```python
from build123d import *

# Parameters (mm, degrees)
SKETCH_1_R               = 3
PLUNGER_1_DEPTH          = 7.4
SKETCH_2_R               = 4.5
RETENTION_FLANGE_2_DEPTH = 1.2


with BuildPart() as part:
    # Эскиз1 → Plunger_1 (new body)
    with BuildSketch(Plane(origin=(0, -68, 0), x_dir=(1, 0, 0), z_dir=(0, 1, 0))):
        with Locations(Location((38, -77, 0), (0, 0, 270))):
            Circle(SKETCH_1_R)
    extrude(amount=PLUNGER_1_DEPTH)

    # Эскиз2 → Retention_flange_2 (add)
    with BuildSketch(Plane(origin=(0, -63.8, 0), x_dir=(1, 0, 0), z_dir=(0, 1, 0))):
        with Locations(Location((38, -77, 0), (0, 0, 270))):
            Circle(SKETCH_2_R)
    extrude(amount=RETENTION_FLANGE_2_DEPTH)


solid = part.part
```
Geometry check sheet. Reference: the model listing, model coordinates, mm. A direction names the side the tool comes from. Give positions to 0.01 mm unless a question says otherwise; leave off trailing zeros. Write each loop counter-clockwise with the first axis right and the second up, starting at its lowest first coordinate (ties: lowest second). Pieces come first, ordered by that corner, then holes. Notation, with made-up numbers: (29, 13) -> (37, 13) arc R21 ccw to (37, 40) -> close; hole circle Ø3 at (30, 28.25). An arc over 180 degrees is marked (long way). Use one line per item in the form item = value.
Item 1: Sectioned sample at C-C on y = -67. Enter the section's corners in (x, z), plus the area to 3 significant figures.
Results list:
outline = circle Ø6 at (38, 77)
area = 28.3 mm2
Item 2: Scan lines: line 1 (Y direction, x = 39, z = 80.75); line 2 (Z direction, x = 38, y = -62.25); line 3 (X direction, y = -61.25, z = 78.75). Record each from-to range of solid material in increasing order.
Results list:
line_1 = -63.8 to -62.6
line_2 = 74 to 80
line_3 = 35.56 to 40.44
Item 3: Sectioned sample at A-A on z = 77. Enter the section's corners in (x, y), plus the area to 3 significant figures.
Results list:
outline = (33.5, -63.8) -> (35, -63.8) -> (35, -68) -> (41, -68) -> (41, -63.8) -> (42.5, -63.8) -> (42.5, -62.6) -> (41, -62.6) -> (41, -60.6) -> (35, -60.6) -> (35, -62.6) -> (33.5, -62.6) -> close
area = 48.0 mm2
Item 4: Depth check by flat-ended pin: pin 1 Ø2 at (y, z) = (-64, 76.5) entering from +X; pin 2 Ø1.5 at (y, z) = (-62.5, 79.5) entering from +X; pin 3 Ø4 at (x, y) = (35.5, -63) entering from +Z; pin 4 Ø3 at (y, z) = (-66, 78) entering from +X. Enter the tip coordinate at first touch or a pass-through.
Results list:
pin_1 = 42.5
pin_2 = 42.14
pin_3 = 81.47
pin_4 = 41
Item 5: Sectioned sample at B-B on x = 38. Enter the section's corners in (y, z), plus the area to 3 significant figures.
Results list:
outline = (-68, 74) -> (-63.8, 74) -> (-63.8, 72.5) -> (-62.6, 72.5) -> (-62.6, 74) -> (-60.6, 74) -> (-60.6, 80) -> (-62.6, 80) -> (-62.6, 81.5) -> (-63.8, 81.5) -> (-63.8, 80) -> (-68, 80) -> close
area = 48.0 mm2
Item 6: Access from +Z, -Z, +X, -X, +Y, -Y to the whole of each face (thin tool, end or side, straight path). Record for faces 1 (the cylindrical face through (33.61, -63.21, 76.02)), 2 (the flat face through (35, -63.8, 78)), 3 (the flat face through (35, -62.6, 78)).
Results list:
face_1 = +Y, -Y
face_2 = -Y
face_3 = +Y
Item 7: Sectioned sample at D-D on z = 73.75. Enter the section's corners in (x, y).
Results list:
outline = (34.89, -63.8) -> (41.11, -63.8) -> (41.11, -62.6) -> (34.89, -62.6) -> close
